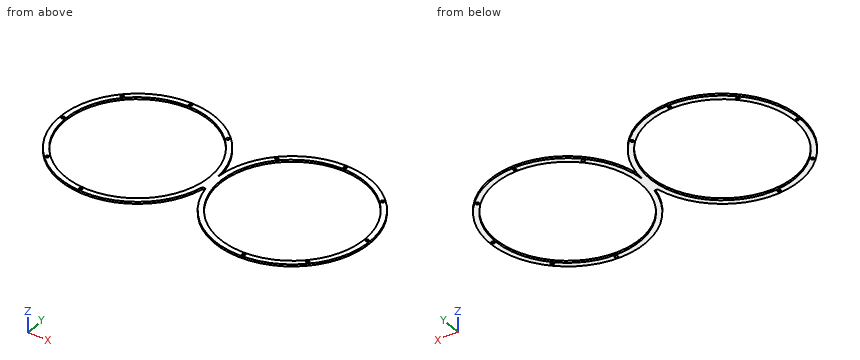
from build123d import *

# Parameters (mm, degrees)
SKETCH_2_R      = 1.5
EXTRUDE_2_DEPTH = 2


with BuildPart() as part:
    # 草图2 → 凸台-拉伸2 (new body)
    with BuildSketch(Plane.XY):
        with BuildLine():
            ThreePointArc((-51.905600365, 30), (-201.574285493, 30.30226796), (-53.265307717, 10.171351817))
            Line((-53.265307717, 10.171351817), (-50.234692283, 10.171351817))
            ThreePointArc((-50.234692283, 10.171351817), (98.074285493, 30.30226796), (-51.594399635, 30))
            Line((-51.594399635, 30), (-51.905600365, 30))
        make_face()
        with Locations((-130.75, -47.218219255)):
            Circle(SKETCH_2_R, mode=Mode.SUBTRACT)
        with Locations((-178.015241636, -26.093889819)):
            Circle(SKETCH_2_R, mode=Mode.SUBTRACT)
        with Locations((27.25, -47.218219255)):
            Circle(SKETCH_2_R, mode=Mode.SUBTRACT)
        with Locations((74.515241636, -26.093889819)):
            Circle(SKETCH_2_R, mode=Mode.SUBTRACT)
        with Locations((-199.25, 25.171351817)):
            Circle(SKETCH_2_R, mode=Mode.SUBTRACT)
        with BuildLine():
            ThreePointArc((-56.757143222, 26.171351817), (-56.751785828, 25.671364573), (-56.75, 25.171351817))
            ThreePointArc((-56.75, 25.171351817), (-56.751785828, 24.671339061), (-56.757143222, 24.171351817))
            ThreePointArc((-56.757143222, 24.171351817), (-62.078432724, -1.616488449), (-76.550469556, -23.613965065))
            ThreePointArc((-76.550469556, -23.613965065), (-77.252525317, -24.326122866), (-77.964683119, -25.028178627))
            ThreePointArc((-77.964683119, -25.028178627), (-99.962159734, -39.500215459), (-125.75, -44.821504962))
            ThreePointArc((-125.75, -44.821504962), (-126.75, -44.828648183), (-127.75, -44.821504962))
            ThreePointArc((-127.75, -44.821504962), (-153.537840266, -39.500215459), (-175.535316881, -25.028178627))
            ThreePointArc((-175.535316881, -25.028178627), (-176.247474683, -24.326122866), (-176.949530444, -23.613965065))
            ThreePointArc((-176.949530444, -23.613965065), (-191.421567276, -1.616488449), (-196.742856778, 24.171351817))
            ThreePointArc((-196.742856778, 24.171351817), (-196.75, 25.171351817), (-196.742856778, 26.171351817))
            ThreePointArc((-196.742856778, 26.171351817), (-191.421567276, 51.959192082), (-176.949530444, 73.956668698))
            ThreePointArc((-176.949530444, 73.956668698), (-176.247474683, 74.6688265), (-175.535316881, 75.370882261))
            ThreePointArc((-175.535316881, 75.370882261), (-153.537840266, 89.842919093), (-127.75, 95.164208595))
            ThreePointArc((-127.75, 95.164208595), (-126.75, 95.171351817), (-125.75, 95.164208595))
            ThreePointArc((-125.75, 95.164208595), (-99.962159734, 89.842919093), (-77.964683119, 75.370882261))
            ThreePointArc((-77.964683119, 75.370882261), (-77.252525317, 74.6688265), (-76.550469556, 73.956668698))
            ThreePointArc((-76.550469556, 73.956668698), (-62.078432724, 51.959192082), (-56.757143222, 26.171351817))
        make_face(mode=Mode.SUBTRACT)
        with Locations((-178.015241636, 76.436593453)):
            Circle(SKETCH_2_R, mode=Mode.SUBTRACT)
        with Locations((-75.484758364, 76.436593453)):
            Circle(SKETCH_2_R, mode=Mode.SUBTRACT)
        with Locations((-126.75, 97.671351817)):
            Circle(SKETCH_2_R, mode=Mode.SUBTRACT)
        with BuildLine():
            ThreePointArc((93.242856778, 26.171351817), (93.248214172, 25.671364573), (93.25, 25.171351817))
            ThreePointArc((93.25, 25.171351817), (93.248214172, 24.671339061), (93.242856778, 24.171351817))
            ThreePointArc((93.242856778, 24.171351817), (87.921567276, -1.616488449), (73.449530444, -23.613965065))
            ThreePointArc((73.449530444, -23.613965065), (72.747474683, -24.326122866), (72.035316881, -25.028178627))
            ThreePointArc((72.035316881, -25.028178627), (50.037840266, -39.500215459), (24.25, -44.821504962))
            ThreePointArc((24.25, -44.821504962), (23.25, -44.828648183), (22.25, -44.821504962))
            ThreePointArc((22.25, -44.821504962), (-3.537840266, -39.500215459), (-25.535316881, -25.028178627))
            ThreePointArc((-25.535316881, -25.028178627), (-26.247474683, -24.326122866), (-26.949530444, -23.613965065))
            ThreePointArc((-26.949530444, -23.613965065), (-41.421567276, -1.616488449), (-46.742856778, 24.171351817))
            ThreePointArc((-46.742856778, 24.171351817), (-46.75, 25.171351817), (-46.742856778, 26.171351817))
            ThreePointArc((-46.742856778, 26.171351817), (-41.421567276, 51.959192082), (-26.949530444, 73.956668698))
            ThreePointArc((-26.949530444, 73.956668698), (-26.247474683, 74.6688265), (-25.535316881, 75.370882261))
            ThreePointArc((-25.535316881, 75.370882261), (-3.537840266, 89.842919093), (22.25, 95.164208595))
            ThreePointArc((22.25, 95.164208595), (23.25, 95.171351817), (24.25, 95.164208595))
            ThreePointArc((24.25, 95.164208595), (50.037840266, 89.842919093), (72.035316881, 75.370882261))
            ThreePointArc((72.035316881, 75.370882261), (72.747474683, 74.6688265), (73.449530444, 73.956668698))
            ThreePointArc((73.449530444, 73.956668698), (87.921567276, 51.959192082), (93.242856778, 26.171351817))
        make_face(mode=Mode.SUBTRACT)
        with Locations((95.75, 25.171351817)):
            Circle(SKETCH_2_R, mode=Mode.SUBTRACT)
        with Locations((-28.015241636, 76.436593453)):
            Circle(SKETCH_2_R, mode=Mode.SUBTRACT)
        with Locations((23.25, 97.671351817)):
            Circle(SKETCH_2_R, mode=Mode.SUBTRACT)
        with Locations((74.515241636, 76.436593453)):
            Circle(SKETCH_2_R, mode=Mode.SUBTRACT)
    extrude(amount=EXTRUDE_2_DEPTH)


solid = part.part
Source: CAD feature listing. Evaluate the final solid. Frame: model axes, mm. Give positions to 0.01 mm unless a question says otherwise; leave off trailing zeros. Write each loop counter-clockwise with the first axis right and the second up, starting at its lowest first coordinate (ties: lowest second). Pieces come first, ordered by that corner, then holes. Notation, with made-up numbers: (38.25, 50.25) -> (59.25, 50.25) arc R30 cw to (59.25, 89.25) -> close; hole circle Ø2 at (-3.5, 89.25). An arc over 180 degrees is marked (long way). Return JSON: item names as keys, results as strings. Group by question number.
1. Section B-B, the plane x = -98. Output: boundary loops of the cut face in (y, z).
2. Section A-A, the plane y = 69.5. Output: boundary loops of the cut face in (x, z).
3. Section C-C, the plane y = 20. Output: boundary loops of the cut face in (x, z).
4. Section D-D, the plane y = 2. Output: boundary loops of the cut face in (x, z), then the cut area to 3 significant figures.
5. Material intervals for line 1 (X direction, y = 28, z = 1.3); line 2 (Y direction, x = -126.75, z = 0.8); line 3 (Y direction, x = -128, z = 0.9), sorted ascending. Write a range as from..to.
6. Pin query (flat end, axial travel): pin 1 Ø5 at (x, y) = (23.25, 97.67) entering from -Z; pin 2 Ø1 at (x, z) = (33, 0.5) entering from -Y. Return the tip coordinate at first contact, or that it passes through.
Determined:
{
 "1": {"outline": "(-44.1, 0) -> (-38.65, 0) -> (-38.65, 2) -> (-44.1, 2) -> close; (88.99, 0) -> (94.44, 0) -> (94.44, 2) -> (88.99, 2) -> close"},
 "2": {"outline": "(-187.25, 0) -> (-180.93, 0) -> (-180.93, 2) -> (-187.25, 2) -> close; (-72.57, 0) -> (-66.25, 0) -> (-66.25, 2) -> (-72.57, 2) -> close; (-37.25, 0) -> (-30.93, 0) -> (-30.93, 2) -> (-37.25, 2) -> close; (77.43, 0) -> (83.75, 0) -> (83.75, 2) -> (77.43, 2) -> close"},
 "3": {"outline": "(-201.57, 0) -> (-196.56, 0) -> (-196.56, 2) -> (-201.57, 2) -> close; (-56.94, 0) -> (-46.56, 0) -> (-46.56, 2) -> (-56.94, 2) -> close; (93.06, 0) -> (98.07, 0) -> (98.07, 2) -> (93.06, 2) -> close"},
 "4": {"outline": "(-198.08, 0) -> (-192.8, 0) -> (-192.8, 2) -> (-198.08, 2) -> close; (-60.7, 0) -> (-55.42, 0) -> (-55.42, 2) -> (-60.7, 2) -> close; (-48.08, 0) -> (-42.8, 0) -> (-42.8, 2) -> (-48.08, 2) -> close; (89.3, 0) -> (94.58, 0) -> (94.58, 2) -> (89.3, 2) -> close", "area": "42.2 mm2"},
 "5": {"line 1": "x = -201.7..-196.69, -56.81..-46.69, 93.19..98.2", "line 2": "y = -49.83..-44.83, 95.17..96.17, 99.17..100.17", "line 3": "y = -49.82..-44.82, 95.16..96.84, 98.5..100.16"},
 "6": {"pin 1": "stops at z = 0", "pin 2": "stops at y = -49.26"}
}
